from build123d import *

# Parameters (mm, degrees)
SKETCH1_R             = 10
BOSS_EXTRUDE1_DEPTH   = 100
BOSS_EXTRUDE1_2_DEPTH = 100
SKETCH2_R             = 75
BOSS_EXTRUDE2_DEPTH   = 10


with BuildPart() as part:
    # Sketch1 → Boss-Extrude1 (new body)
    with BuildSketch(Plane(origin=(0, 0, 0), x_dir=(1, 0, 0), z_dir=(0, 1, 0))):
        with Locations(Location((30, 30, 0), (0, 0, 270))):
            Circle(SKETCH1_R)
    extrude(amount=BOSS_EXTRUDE1_DEPTH)


with BuildPart() as body_2:
    # Sketch1 → Boss-Extrude1 2 (new body)
    with BuildSketch(Plane(origin=(0, 0, 0), x_dir=(1, 0, 0), z_dir=(0, 1, 0))):
        with Locations(Location((30, -30, 0), (0, 0, 90))):
            Circle(SKETCH1_R)
    extrude(amount=BOSS_EXTRUDE1_2_DEPTH)


with BuildPart() as body_3:
    # Mirror1: mirrored copy
    add(body_2.part.mirror(Plane(origin=(0, 0, 0), x_dir=(0, 0, 1), z_dir=(1, 0, 0))))


with BuildPart() as body_4:
    # Mirror1 2: mirrored copy
    add(part.part.mirror(Plane(origin=(0, 0, 0), x_dir=(0, 0, 1), z_dir=(1, 0, 0))))


with BuildPart() as part_1:
    add(part.part)

    add(body_2.part)  # Boss-Extrude2 merges body 2

    add(body_3.part)  # Boss-Extrude2 merges body 3

    add(body_4.part)  # Boss-Extrude2 merges body 4
    # Sketch2 → Boss-Extrude2 (add)
    with BuildSketch(Plane(origin=(0, 100, 0), x_dir=(1, 0, 0), z_dir=(0, 1, 0))):
        with Locations(Location((0, 0, 0), (0, 0, 270))):
            Circle(SKETCH2_R)
    extrude(amount=-BOSS_EXTRUDE2_DEPTH)


solid = part_1.part
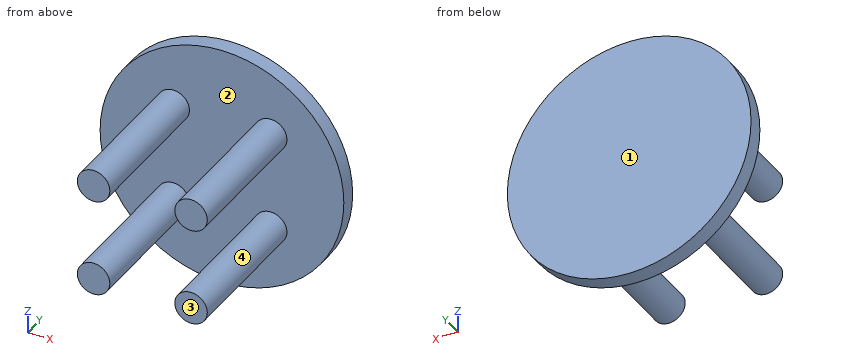
Can you work these out from the model? Positions are in its coordinate system, mm. Face numbers are marked on the shaded views. A direction names the side the tool comes from. Coordinates: 2 decimals unless noted, no trailing zeros. Order: outer loops, then holes, each group sorted by start corner. A loop starts at its lowest first (then second) coordinate and runs counter-clockwise, first axis right, second up. Notation, with made-up numbers: (-35, -25) - (4, -25) arc R19 cw to (4, 2) - close; hole circle Ø2 at (76.25, -6.75). An arc over 180 degrees is marked (long way). Answer as a JSON object with one key per item and string values. Group by question number.
Q1. On a 3-axis mill with a long thin cutter (end or side, diameter ignored), from which of +Z, -Z, +X, -X, +Y, -Y can I reach the whole of each face in a straight line? I mean the marked faces 1 and 2. Say none if no direction works.
Q2. Imagine slicing it at B-B (x = 30). Please give me the cut outline in (y, z), and give its area (3 significant figures).
Q3. Imagine slicing it at D-D (x = 0). Please give me the cut outline in (y, z), and give its area (3 significant figures).
Q4. Will these pins go through, and if not, where does the flat tip stop? P1, Ø6, axis at x = -21, y = 62.5, coming from the +Z side; P2, Ø1, axis at x = -29.5, y = 58.5, coming from the -Z side.
Q5. Imagine slicing it at C-C (z = -30). Please give me the cut outline in (x, y), and give its area (3 significant figures).
Q6. I need wall thicknesses on line 1 (Y direction, x = -24, z = -44); line 2 (Z direction, x = 29, y = 66); line 3 (X direction, y = 58.5, z = 28.5). Which ranges of each line are inside material? Lowest first, please. Write a range as from..to.
Q7. We'd pull the mould along X, two halves only. Please class the marked faces 3 and 4: +X half, -X half, draft (parallel to the pull), parting line (faces both ways), or undercut.
Q8. Imagine slicing it at A-A (y = 22). Please give me the cut outline in (x, z).
Determined:
{
 "1": {"face 1": "+Z, -Z, +X, -X, +Y", "face 2": "-Y"},
 "2": {"outline": "(0, -40) - (90, -40) - (90, -68.74) - (100, -68.74) - (100, 68.74) - (90, 68.74) - (90, 40) - (0, 40) - (0, 20) - (90, 20) - (90, -20) - (0, -20) - close", "area": "4,970 mm2"},
 "3": {"outline": "(90, -75) - (100, -75) - (100, 75) - (90, 75) - close", "area": "1,500 mm2"},
 "4": {"P1": "stops at z = 38", "P2": "stops at z = -40"},
 "5": {"outline": "(-68.74, 90) - (-40, 90) - (-40, 0) - (-20, 0) - (-20, 90) - (20, 90) - (20, 0) - (40, 0) - (40, 90) - (68.74, 90) - (68.74, 100) - (-68.74, 100) - close", "area": "4,970 mm2"},
 "6": {"line 1": "y = 90..100", "line 2": "z = -39.95..-20.05, 20.05..39.95", "line 3": "x = -39.89..-20.11, 20.11..39.89"},
 "7": {"face 3": "draft", "face 4": "undercut"},
 "8": {"outline": "circle Ø20 at (-30, -30); circle Ø20 at (-30, 30); circle Ø20 at (30, -30); circle Ø20 at (30, 30)"}
}
